from build123d import *

# Parameters (mm, degrees)
F1_DEPTH    = 8
F2_T1_DEPTH = 11.6003561832
F2_T3_DEPTH = 11.8663751546
F2_T5_DEPTH = 11.4631685347
F3_SIZE     = 0.4


# Not quite as in the source:
# - a fillet or chamfer that OpenCascade refuses, or shapes differently, is made with other operations: its cross-section is extruded or revolved along the edge and cut away or added


with BuildPart() as f1:
    # F0 (on Top) → F1 (new body)
    with BuildSketch(Plane.XY):
        with BuildLine():
            Line((-21, 8), (-19, 8))
            Line((-19, 8), (-19, 18))
            Line((-19, 18), (-10, 18))
            Line((-10, 18), (-10, 0))
            ThreePointArc((-10, 0), (0, -10), (10, 0))
            Line((10, 0), (8, 0))
            ThreePointArc((8, 0), (0, -8), (-8, 0))
            Line((-8, 0), (-8, 20))
            Line((-8, 20), (-21, 20))
            Line((-21, 20), (-21, 8))
        make_face()
    extrude(amount=F1_DEPTH)

    # F2: chamfer of 0.7 on 6 edges, made by hand

    # F2_s2 → F2_t1 (cut)
    with BuildSketch(Plane.XY.offset(-1.8001780916)):
        Polygon((-8, 19.3), (-8.7, 20), (-8, 20), align=None)
        Polygon((-20.3, 20), (-21, 19.3), (-21, 20), align=None)
        Polygon((-20.3, 8), (-21, 8.7), (-21, 8), align=None)
        Polygon((-19.7, 8), (-19, 8.7), (-19, 8), align=None)
    extrude(amount=F2_T1_DEPTH, mode=Mode.SUBTRACT)

    # F2_s4 → F2_t3 (cut)
    with BuildSketch(Plane.XY.offset(-1.9331875773)):
        with BuildLine():
            Line((9.9716327909, -0.752688172), (9.2736184955, 0))
            Line((9.2736184955, 0), (10, 0))
            ThreePointArc((10, 0), (9.9925280661, -0.3865007745), (9.9716327909, -0.752688172))
        make_face()
    extrude(amount=F2_T3_DEPTH, mode=Mode.SUBTRACT)

    # F2_s6 → F2_t5 (cut)
    with BuildSketch(Plane.XY.offset(-1.7315842673)):
        with BuildLine():
            Line((8.6717933555, 0), (7.9740628556, -0.6436781609))
            ThreePointArc((7.9740628556, -0.6436781609), (7.9931075422, -0.332011775), (8, 0))
            Line((8, 0), (8.6717933555, 0))
        make_face()
    extrude(amount=F2_T5_DEPTH, mode=Mode.SUBTRACT)

    # F3
    f3_edges = [f1.edges().sort_by_distance(p)[0] for p in [
        (-20.65, 19.65, 8),
        (-14.5, 20, 8),
        (-8.35, 19.65, 8),
        (-8, 9.65, 8),
        (-0.3221, -7.993513, 8),
        (8.322928, -0.321839, 8),
        (8.972706, 0, 8),
        (9.622626, -0.376344, 8),
        (-0.376611, -9.992906, 8),
        (-10, 9, 8),
        (-14.5, 18, 8),
        (-19, 13.35, 8),
        (-19.35, 8.35, 8),
        (-20, 8, 8),
        (-20.65, 8.35, 8),
        (-21, 14, 8),
        (-20.65, 19.65, 0),
        (-14.5, 20, 0),
        (-8.35, 19.65, 0),
        (-8, 9.65, 0),
        (-0.3221, -7.993513, 0),
        (8.322928, -0.321839, 0),
        (8.972706, 0, 0),
        (9.622626, -0.376344, 0),
        (-0.376611, -9.992906, 0),
        (-10, 9, 0),
        (-14.5, 18, 0),
        (-19, 13.35, 0),
        (-19.35, 8.35, 0),
        (-20, 8, 0),
        (-20.65, 8.35, 0),
        (-21, 14, 0),
    ]]
    chamfer(f3_edges, length=F3_SIZE)


solid = f1.part
Design review of the part built by this model. Coordinates are the model's own, in mm. A direction names the side the tool comes from. Coordinates: 2 decimals unless noted, no trailing zeros. Order: outer loops, then holes, each group sorted by start corner. A loop starts at its lowest first (then second) coordinate and runs counter-clockwise, first axis right, second up. Notation, with made-up numbers: (43, 27.5) -> (50, 27.5) arc R23 ccw to (50, 48.5) -> close; hole circle Ø11 at (86, 59.25). An arc over 180 degrees is marked (long way). One line per item, written item: value.
1) Draft analysis for pull direction X (two halves, no side actions). For faces 1 (the face through (-9, 5, 0)), 2 (the face through (-19, 13, 4)), 3 (the face through (8.452, -0.471, 0.203)), 4 (the face through (-0.574, -9.697, 0.114)), state which applies: +X half, -X half, draft (parallel to the pull), parting line (faces both ways), or undercut.
Output values:
face 1: draft
face 2: undercut
face 3: undercut
face 4: parting line
2) We need section A-A, the plane x = 0. Give the boundary of the cut face in (y, z), then the cut area to 3 significant figures.
Output values:
outline: (-10, 0.4) -> (-9.6, 0) -> (-8.4, 0) -> (-8, 0.4) -> (-8, 7.6) -> (-8.4, 8) -> (-9.6, 8) -> (-10, 7.6) -> close
area: 15.7 mm2
3) Machinability: for faces 5 (the face through (8.452, -0.471, 7.797)), 6 (the face through (-8.494, 19.515, 0.203)), 7 (the face through (-19.489, 8.498, 7.803)), which of the approach directions +Z, -Z, +X, -X, +Y, -Y give a long, thin tool a straight path to every point of the face, cutting with its end or side? Answer none if there is none.
Output values:
face 5: +Z, +Y
face 6: -Z, +X, +Y
face 7: +Z, -Y
4) We need section B-B, the plane z = 5. Give the boundary of the cut face in (x, y).
Output values:
outline: (-21, 8.7) -> (-20.3, 8) -> (-19.7, 8) -> (-19, 8.7) -> (-19, 18) -> (-10, 18) -> (-10, 0) arc R10 ccw to (9.97, -0.75) -> (9.27, 0) -> (8.67, 0) -> (7.97, -0.64) arc R8 cw to (-8, 0) -> (-8, 19.3) -> (-8.7, 20) -> (-20.3, 20) -> (-21, 19.3) -> close
5) To check wall thickness, follow probe 1 along X at (y, z) = (15.25, 2.5); probe 2 along Y at (x, z) = (-10.5, 2); probe 3 along Y at (x, z) = (0, 1.25). State the ranges of each line that lie inside material, in increasing order. Write a range as [from, to].
Output values:
probe 1: x = [-21, -19], [-10, -8]
probe 2: y = [18, 20]
probe 3: y = [-10, -8]
6) Clearance check with flat-ended pins moving along their axes: P1, Ø10, axis at x = -15.5, y = -6.5, coming from the +Z side; P2, Ø3.5, axis at x = -14, z = 5.5, coming from the -Y side; P3, Ø2, axis at y = 7.5, z = 6.5, coming from the +X side; P4, Ø3, axis at x = 6.5, z = 5.5, coming from the -Y side. State where each tip first meets the part, or that it passes through.
Output values:
P1: passes through
P2: stops at y = 18
P3: stops at x = -8
P4: stops at y = -8.66
